```python
from build123d import *

# Parameters (mm, degrees)
CYLINDER_R           = 10
CYLINDER_DEPTH       = 1000
CYLINDER_PITCH_ANGLE = 90


with BuildPart() as part:
    # Cylinder → Cylinder (new body)
    with BuildSketch(Plane.XY):
        Circle(CYLINDER_R)
    extrude(amount=CYLINDER_DEPTH)


with BuildPart() as part_1:
    # Cylinder pitch: moved
    add(part.part.rotate(Axis((0, 0, 0), (0, 1, 0)), CYLINDER_PITCH_ANGLE))


with BuildPart() as part_2:
    # Cylinder placement: moved
    add(part_1.part.moved(Location((-500, 0, 0))))


solid = part_2.part
```
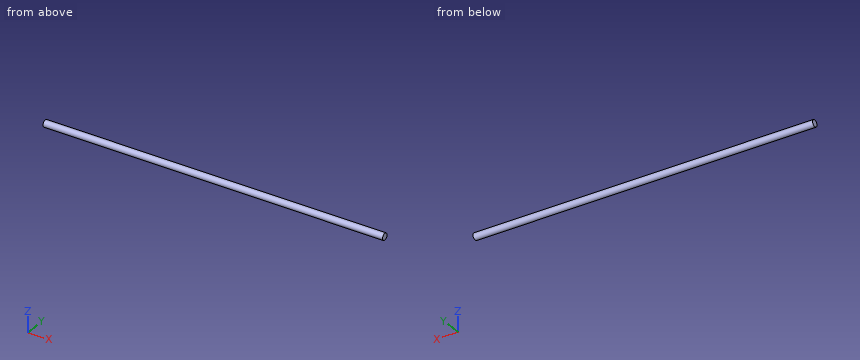
The listing builds one solid part. Answer for the finished solid, in the listing's coordinates (mm). Coordinates: 2 decimals unless noted, no trailing zeros. Write each loop counter-clockwise with the first axis right and the second up, starting at its lowest first coordinate (ties: lowest second). Pieces come first, ordered by that corner, then holes. Notation, with made-up numbers: M 4.5,56 L 26.5,56 A19 ccw 26.5,62 Z; hole C 16,88 d9. An arc over 180 degrees is marked long. Use a Markdown table: item, result. Add a question column.
1. Section B-B (z = -3.5) is taken. Give the vertices of the cut face in (x, y).
2. Given P1, Ø10, axis at x = 362, z = 3.5, coming from the -Y side; P2, Ø10, axis at x = -323, z = -7, coming from the -Y side; P3, Ø4, axis at x = -80, y = 7, coming from the -Z side; P4, Ø1, axis at x = -221.5, y = -6.5, coming from the +Z side, each flat-ended and moving along its own axis, determine where each tip first touches the part or whether it passes through.
3. Straight lines are drawn through the part: line 1 along Y through (x, z) = (252.5, 0.75); line 2 along Z through (x, y) = (-297, -8); line 3 along Y through (x, z) = (41, -4). For each, find the intervals that lie inside material, in ascending order. Write a range as [from, to].
4. Section C-C (y = 6.25) is taken. Give the vertices of the cut face in (x, z).
5. Section A-A (x = -263.5) is taken. Give the vertices of the cut face in (y, z).
Data:
| question | item | result |
|---|---|---|
| 1 | outline | M -500,-9.37 L 500,-9.37 L 500,9.37 L -500,9.37 Z |
| 2 | P1 | stops at y = -10 |
| 2 | P2 | stops at y = -9.8 |
| 2 | P3 | stops at z = -8.66 |
| 2 | P4 | stops at z = 8 |
| 3 | line 1 | y = [-9.97, 9.97] |
| 3 | line 2 | z = [-6, 6] |
| 3 | line 3 | y = [-9.17, 9.17] |
| 4 | outline | M -500,-7.81 L 500,-7.81 L 500,7.81 L -500,7.81 Z |
| 5 | outline | C 0,0 d20 |
